from build123d import *

# Parameters (mm, degrees)
F0_W      = 37.084
F0_H      = 30.734
F0_W_2    = 26.416
F0_H_2    = 20.066
F1_DEPTH  = 15.875
F2_W      = 12.192
F2_H      = 5.842
F3_DEPTH  = 31.75
F4_W      = 82.55
F4_H      = 12.7
F5_DEPTH  = 19.05
F7_DEPTH  = 6.35
F9_R      = 3
F10_DEPTH = 30.735


with BuildPart() as f1:
    # F0 (on Top) → F1 (new body, symmetric)
    with BuildSketch(Plane.XY):
        Rectangle(F0_W, F0_H)
        Rectangle(F0_W_2, F0_H_2, mode=Mode.SUBTRACT)
    extrude(amount=F1_DEPTH, both=True)

    # F2 (on face) → F3 (join)
    with BuildSketch(Plane.XY.offset(15.875)):
        with Locations((0, 7.112)):
            Rectangle(F2_W, F2_H)
    extrude(amount=-F3_DEPTH)

    # F4 (on face) → F5 (join)
    with BuildSketch(Plane(origin=(0, 0, -15.875), x_dir=(1, 0, 0), z_dir=(0, 0, -1))):
        with Locations((59.817, 9.017)):
            Rectangle(F4_W, F4_H)
    extrude(amount=-F5_DEPTH)

    # F6 (on face) → F7 (join)
    with BuildSketch(Plane.XZ.offset(15.367)):
        Polygon((43.942, 3.175), (18.542, 15.875), (18.542, 3.175), align=None)
    extrude(amount=-F7_DEPTH)

    # F9 (on face) → F10 (cut, through all)
    with BuildSketch(Plane.XZ.offset(15.367)):
        Circle(F9_R)
    extrude(amount=-F10_DEPTH, mode=Mode.SUBTRACT)


solid = f1.part
For this review, take the finished solid that the model builds, in its own axes (mm). A direction names the side the tool comes from. Round coordinates to 2 decimals unless told otherwise and drop trailing zeros. Order: outer loops, then holes, each group sorted by start corner. A loop starts at its lowest first (then second) coordinate and runs counter-clockwise, first axis right, second up. Notation, with made-up numbers: M -27,-25 L -10,-25 A26 cw -10,-5 Z; hole C 43,-24 d6. An arc over 180 degrees is marked long. Use a Markdown table: item, result. Add a question column.
Item 1: Mouldability with a two-part tool opening along Y and no side actions: class faces 1 (the flat face through (-13.208, 0, 0)), 2 (the flat face through (59, -2.667, -6)), 3 (the flat face through (0, 7, 15.875)), 4 (the flat face through (6.096, 7, 0)) as released by +Y, released by -Y, zero draft, split by the parting line, or undercut.
Item 2: Add section B-B, the plane z = 0. Give the boundary of the cut face in (x, y).
Item 3: Add section A-A, the plane y = 9. Give the boundary of the cut face in (x, z) (3 decimals), then the cut area to 3 significant figures.
Item 4: Tool access review of faces 5 (the flat face through (10, 10.033, 0)), 6 (the flat face through (0, 15.367, 4)), 7 (the flat face through (25, -9.017, 7)): name each direction out of +Z, -Z, +X, -X, +Y, -Y from which nothing blocks a thin tool from reaching the whole face with its end or side.
Item 5: Insertion check: pin 1 (5.5 mm diameter, centred on x = 43.5, z = -7, fed in from +Y); pin 2 (6.5 mm diameter, centred on x = 25, z = 10, fed in from +Y); pin 3 (3 mm diameter, centred on y = 7.5, z = -7.5, fed in from +X). Each pin has a flat end and moves straight along its axis. Give the tip position at first contact, or say it passes through.
Item 6: To check wall thickness, follow line 1 along X through (y, z) = (6.5, -3.5); line 2 along X through (y, z) = (-3.5, -7); line 3 along X through (y, z) = (3, 12). State the ranges of each line that lie inside material, in increasing order.
Item 7: Add section D-D, the plane x = 0. Give the boundary of the cut face in (y, z) (3 decimals), then the cut area to 3 significant figures.
Item 8: Add section C-C, the plane y = 3. Give the boundary of the cut face in (x, z) (3 decimals), then the cut area to 3 significant figures.
Geometry results:
| question | item | result |
|---|---|---|
| 1 | face 1 | undercut |
| 1 | face 2 | released by +Y |
| 1 | face 3 | zero draft |
| 1 | face 4 | undercut |
| 2 | outline | M -18.54,-15.37 L -3,-15.37 L -3,-10.03 L -13.21,-10.03 L -13.21,10.03 L -6.1,10.03 L -6.1,4.19 L -3,4.19 L -3,15.37 L -18.54,15.37 Z; M 3,-15.37 L 101.09,-15.37 L 101.09,-2.67 L 18.54,-2.67 L 18.54,15.37 L 3,15.37 L 3,4.19 L 6.1,4.19 L 6.1,10.03 L 13.21,10.03 L 13.21,-10.03 L 3,-10.03 Z |
| 3 | outline | M -18.542,-15.875 L -13.208,-15.875 L -13.208,15.875 L -18.542,15.875 Z; M -6.096,-15.875 L 6.096,-15.875 L 6.096,15.875 L -6.096,15.875 Z; M 13.208,-15.875 L 18.542,-15.875 L 18.542,15.875 L 13.208,15.875 Z; hole C 0,0 d6 |
| 3 | area | 698 mm² |
| 4 | face 5 | +Z, -Z |
| 4 | face 6 | +Z, -Z, +X, -X, +Y |
| 4 | face 7 | +Z, +X, +Y |
| 5 | pin 1 | stops at y = -2.67 |
| 5 | pin 2 | stops at y = -9.02 |
| 5 | pin 3 | stops at x = 18.54 |
| 6 | line 1 | x = -18.54 to -13.21, -6.1 to 6.1, 13.21 to 18.54 |
| 6 | line 2 | x = -18.54 to -13.21, 13.21 to 101.09 |
| 6 | line 3 | x = -18.54 to -13.21, 13.21 to 18.54 |
| 7 | outline | M -15.367,-15.875 L -10.033,-15.875 L -10.033,-3 L -15.367,-3 Z; M -15.367,3 L -10.033,3 L -10.033,15.875 L -15.367,15.875 Z; M 4.191,-15.875 L 15.367,-15.875 L 15.367,-3 L 4.191,-3 Z; M 4.191,3 L 15.367,3 L 15.367,15.875 L 4.191,15.875 Z |
| 7 | area | 425 mm² |
| 8 | outline | M -18.542,-15.875 L -13.208,-15.875 L -13.208,15.875 L -18.542,15.875 Z; M 13.208,-15.875 L 18.542,-15.875 L 18.542,15.875 L 13.208,15.875 Z |
| 8 | area | 339 mm² |
